```python
from build123d import *

# Parameters (mm, degrees)
SKETCH1_R           = 2
BOSS_EXTRUDE1_DEPTH = 98
SKETCH2_R           = 2.75
BOSS_EXTRUDE2_DEPTH = 1
BOSS_EXTRUDE3_START = 1
SKETCH3_R           = 2.75
BOSS_EXTRUDE3_DEPTH = 1
CUT_EXTRUDE1_DEPTH  = 0.5
CUT_EXTRUDE2_DEPTH  = 0.5


with BuildPart() as part:
    # Sketch1 → Boss-Extrude1 (new body)
    with BuildSketch(Plane.XY):
        Circle(SKETCH1_R)
    extrude(amount=BOSS_EXTRUDE1_DEPTH)

    # Sketch2 → Boss-Extrude2 (add)
    with BuildSketch(Plane.XY.offset(98)):
        Circle(SKETCH2_R)
    extrude(amount=BOSS_EXTRUDE2_DEPTH)

    # Sketch3 → Boss-Extrude3 (add)
    with BuildSketch(Plane(origin=(0, 0, 0), x_dir=(-1, 0, 0), z_dir=(0, 0, -1)).offset(BOSS_EXTRUDE3_START)):
        with Locations(Location((0, 0, 0), (0, 0, 180))):
            Circle(SKETCH3_R)
    extrude(amount=-BOSS_EXTRUDE3_DEPTH)

    # Sketch4 → Cut-Extrude1 (cut)
    with BuildSketch(Plane(origin=(0, 0, -1), x_dir=(-1, 0, 0), z_dir=(0, 0, -1))):
        Polygon((-0.154926193, -0.160877279), (-0.154926193, -2.234675522), (0.154926193, -2.234675522), (0.154926193, -0.160877279), (2.234675522, -0.160877279), (2.234675522, 0.160877279), (0.154926193, 0.160877279), (0.154926193, 2.234675522), (-0.154926193, 2.234675522), (-0.154926193, 0.160877279), (-2.234675522, 0.160877279), (-2.234675522, -0.160877279), align=None)
    extrude(amount=-CUT_EXTRUDE1_DEPTH, mode=Mode.SUBTRACT)

    # Sketch5 → Cut-Extrude2 (cut)
    with BuildSketch(Plane.XY.offset(99)):
        Polygon((-2.234675522, -0.160877279), (-0.154926193, -0.160877279), (-0.154926193, -2.234675522), (0.154926193, -2.234675522), (0.154926193, -0.160877279), (2.234675522, -0.160877279), (2.234675522, 0.160877279), (0.154926193, 0.160877279), (0.154926193, 2.234675522), (-0.154926193, 2.234675522), (-0.154926193, 0.160877279), (-2.234675522, 0.160877279), align=None)
    extrude(amount=-CUT_EXTRUDE2_DEPTH, mode=Mode.SUBTRACT)


solid = part.part
```
Design review of the part built by this model. Coordinates are the model's own, in mm. A direction names the side the tool comes from. Round coordinates to 2 decimals unless told otherwise and drop trailing zeros. Write each loop counter-clockwise with the first axis right and the second up, starting at its lowest first coordinate (ties: lowest second). Pieces come first, ordered by that corner, then holes.
Item 1: We need section B-B on x = -1.05. Write out the cut boundary in (y, z), and give its area (3 significant figures).
Item 2: For probe 1 along Z at (x, y) = (2.1, -0.05); probe 2 along Z at (x, y) = (-0.05, 0.3); probe 3 along Z at (x, y) = (1.4, 2.15), list the stretches that pass through material, from the lowest coordinate up.
Item 3: Clearance check with flat-ended pins moving along their axes: pin 1 Ø0.6 at (y, z) = (-0.5, 98.5) entering from -X; pin 2 Ø1.5 at (y, z) = (2, 40.5) entering from +X; pin 3 Ø3 at (x, y) = (0, -0.5) entering from +Z; pin 4 Ø3 at (y, z) = (-2, 75.5) entering from -X. State where each tip first meets the part, or that it passes through.
Item 4: For faces 5 (the flat face through (1, -2, 98)), 6 (the cylindrical face through (-0.596, -2.685, 98.493)), list the 3-axis set-ups (+Z, -Z, +X, -X, +Y, -Y) from which the entire face can be reached by the end or side of a thin tool; tool diameter is ignored.
Item 5: We need section C-C on z = 15.5. Write out the cut boundary in (x, y), and give its area (3 significant figures).
Item 6: We need section A-A on y = 1. Write out the cut boundary in (x, z), and give its area (3 significant figures).
Item 7: The part is to be moulded in two halves that separate along X. For faces 1 (the cylindrical face through (0, -2, 48)), 2 (the flat face through (1, 2, 0)), 3 (the flat face through (0, 0, -0.5)), 4 (the flat face through (0, 0, 98.5)), say which applies: +X half, -X half, draft (parallel to the pull), parting line (faces both ways), or undercut.
Returned:
1. outline: (-2.54, -1) - (-0.16, -1) - (-0.16, -0.5) - (0.16, -0.5) - (0.16, -1) - (2.54, -1) - (2.54, 0) - (1.7, 0) - (1.7, 98) - (2.54, 98) - (2.54, 99) - (0.16, 99) - (0.16, 98.5) - (-0.16, 98.5) - (-0.16, 99) - (-2.54, 99) - (-2.54, 98) - (-1.7, 98) - (-1.7, 0) - (-2.54, 0) - close
1. area: 343 mm2
2. probe 1: z = -0.5 to 0, 98 to 98.5
2. probe 2: z = -0.5 to 98.5
2. probe 3: z = -1 to 0, 98 to 99
3. pin 1: stops at x = -2.74
3. pin 2: stops at x = 1.56
3. pin 3: stops at z = 99
3. pin 4: stops at x = -1.94
4. face 5: none
4. face 6: +Z, -Z
5. outline: circle Ø4 at (0, 0)
5. area: 12.6 mm2
6. outline: (-2.56, -1) - (-0.15, -1) - (-0.15, -0.5) - (0.15, -0.5) - (0.15, -1) - (2.56, -1) - (2.56, 0) - (1.73, 0) - (1.73, 98) - (2.56, 98) - (2.56, 99) - (0.15, 99) - (0.15, 98.5) - (-0.15, 98.5) - (-0.15, 99) - (-2.56, 99) - (-2.56, 98) - (-1.73, 98) - (-1.73, 0) - (-2.56, 0) - close
6. area: 349 mm2
7. face 1: parting line
7. face 2: draft
7. face 3: undercut
7. face 4: undercut
